Can you work these out from the model? Positions are in its coordinate system, mm. Round coordinates to 2 decimals unless told otherwise and drop trailing zeros. Loops run counter-clockwise (first coordinate to the right, second up) from the corner with the lowest first, then second, coordinate; pieces in that order, holes last. Notation, with made-up numbers: (25, 50) - (40, 50) arc R7 cw to (40, 59) - close; hole circle Ø11 at (-29, 38). An arc over 180 degrees is marked (long way). Answer as CSV lines item,"result".
```python
from build123d import *

# Parameters (mm, degrees)
SKETCH_1_R          = 29
EXTRUDE_1_DEPTH     = 6
SKETCH_2_R          = 6.6
CUT_EXTRUDE_1_DEPTH = 42.448763552
SKETCH_3_W          = 1.470113788
SKETCH_3_H          = 15.681213729
CUT_EXTRUDE_2_DEPTH = 42.448763552


with BuildPart() as part:
    # 草图1 → 凸台-拉伸1 (new body)
    with BuildSketch(Plane.XY):
        Circle(SKETCH_1_R)
    extrude(amount=EXTRUDE_1_DEPTH)

    # 草图2 → 切除-拉伸1 (cut, through all)
    with BuildSketch(Plane.XY.offset(6)):
        Circle(SKETCH_2_R)
    extrude(amount=-CUT_EXTRUDE_1_DEPTH, mode=Mode.SUBTRACT)

    # 草图3 → 切除-拉伸2 (cut, through all)
    with BuildSketch(Plane.XY.offset(6)):
        Polygon((15.816409823, 19.992808752), (5.736719933, 7.980302113), (6.86289243, 7.035331186), (16.94258232, 19.047837825), align=None)
        with Locations((0, 17.641365445)):
            Rectangle(SKETCH_3_W, SKETCH_3_H)
        Polygon((24.967202603, 5.148787783), (9.524221746, 2.425773595), (9.779504326, 0.97799414), (25.222485183, 3.701008327), align=None)
        Polygon((22.435563806, -12.104408212), (8.855234354, -4.263801347), (8.120177461, -5.536957234), (21.700506913, -13.377564098), align=None)
        Polygon((9.406075361, -23.693817079), (4.042784393, -8.958296253), (2.661329316, -9.461104781), (8.024620283, -24.196625607), align=None)
        Polygon((-8.024620283, -24.196625607), (-2.661329316, -9.461104781), (-4.042784393, -8.958296253), (-9.406075361, -23.693817079), align=None)
        Polygon((-21.700506913, -13.377564098), (-8.120177461, -5.536957234), (-8.855234354, -4.263801347), (-22.435563806, -12.104408212), align=None)
        Polygon((-25.222485183, 3.701008327), (-9.779504326, 0.97799414), (-9.524221746, 2.425773595), (-24.967202603, 5.148787783), align=None)
        Polygon((-16.94258232, 19.047837825), (-6.86289243, 7.035331186), (-5.736719933, 7.980302113), (-15.816409823, 19.992808752), align=None)
    extrude(amount=-CUT_EXTRUDE_2_DEPTH, mode=Mode.SUBTRACT)


solid = part.part
```
Q1. We'd pull the mould along X, two halves only. Please class faces 1 (the cylindrical face through (13.38, -25.73, 2.96)), 2 (the flat face through (-7, 0, 6)), 3 (the flat face through (-3.342, -9.213, 3.042)): pulls with the +X half, pulls with the -X half, needs draft (parallel to the pull), parting line crosses it, or undercut.
Checks:
face 1,"parting line crosses it"
face 2,"needs draft"
face 3,"undercut"
Q2. Imagine slicing it at A-A (y = 0). Write out the boundary of the cut face in (x, z), then the cut area to 3 significant figures.
Checks:
outline,"(-29, 0) - (-6.6, 0) - (-6.6, 6) - (-29, 6) - close; (6.6, 0) - (29, 0) - (29, 6) - (6.6, 6) - close"
area,"269 mm²"
Q3. Imagine slicing it at D-D (y = -10.5). Write out the boundary of the cut face in (x, z).
Checks:
outline,"(-27.03, 0) - (-19.66, 0) - (-19.66, 6) - (-27.03, 6) - close; (-16.72, 0) - (-4.6, 0) - (-4.6, 6) - (-16.72, 6) - close; (-3.04, 0) - (3.04, 0) - (3.04, 6) - (-3.04, 6) - close; (4.6, 0) - (16.72, 0) - (16.72, 6) - (4.6, 6) - close; (19.66, 0) - (27.03, 0) - (27.03, 6) - (19.66, 6) - close"
Q4. Imagine slicing it at C-C (x = -13.5). Write out the boundary of the cut face in (y, z), then the cut area to 3 significant figures.
Checks:
outline,"(-25.67, 0) - (-8.64, 0) - (-8.64, 6) - (-25.67, 6) - close; (-6.95, 0) - (1.63, 0) - (1.63, 6) - (-6.95, 6) - close; (3.13, 0) - (14.95, 0) - (14.95, 6) - (3.13, 6) - close; (17.23, 0) - (25.67, 0) - (25.67, 6) - (17.23, 6) - close"
area,"275 mm²"
Q5. If I drill on line 1 along Y through (x, z) = (0, 3.35); line 2 along X through (y, z) = (-20, 4); line 3 along X through (y, z) = (11.5, 0.5), over which ranges is the centre line in solid material (lowest first)? Write a range as [from, to].
Checks:
line 1,"[-29, -6.6], [6.6, 9.8], [25.48, 29]"
line 2,"[-21, -8.06], [-6.5, 6.5], [8.06, 21]"
line 3,"[-26.62, -10.61], [-8.69, -0.74], [0.74, 8.69], [10.61, 26.62]"
Q6. Imagine slicing it at B-B (x = 0). Write out the boundary of the cut face in (y, z), then the cut area to 3 significant figures.
Checks:
outline,"(-29, 0) - (-6.6, 0) - (-6.6, 6) - (-29, 6) - close; (6.6, 0) - (9.8, 0) - (9.8, 6) - (6.6, 6) - close; (25.48, 0) - (29, 0) - (29, 6) - (25.48, 6) - close"
area,"175 mm²"
Q7. I'm going to push flat-ended pins straight in: pin 1 Ø1.5 at (x, z) = (-16, 5) entering from +Y; pin 2 Ø3 at (y, z) = (20, 1.5) entering from -X; pin 3 Ø1.2 at (x, z) = (-0.5, 2) entering from -Y. Where does each tip first touch, or does it pass through?
Checks:
pin 1,"y = 24.67"
pin 2,"x = -22.33"
pin 3,"y = -29"
